Geometry check sheet. Reference: the model listing, model coordinates, mm. Coordinates: 2 decimals unless noted, no trailing zeros. Write each loop counter-clockwise with the first axis right and the second up, starting at its lowest first coordinate (ties: lowest second). Pieces come first, ordered by that corner, then holes. Notation, with made-up numbers: M 12,-39 L 39,-39 A18 ccw 39,-18 Z; hole C 33.5,88.5 d8. An arc over 180 degrees is marked long. Put each result on its own line as item: value. Start each with the question number.
1) Cross-section at B-B on z = 22. Record the cut outline in (x, y).
2) Scan lines: line 1 along X through (y, z) = (-6.5, 29); line 2 along X through (y, z) = (-5.75, 8); line 3 along Z through (x, y) = (1.5, -2.75). Record each from-to range of solid material in increasing order.
3) Gauge pin test, flat ends, axial feed: pin 1 (3 mm diameter, centred on x = 6, y = -5, fed in from +Z); pin 2 (10 mm diameter, centred on y = -4, z = 19.5, fed in from +X); pin 3 (5 mm diameter, centred on x = -1, y = -15, fed in from -Z); pin 4 (6 mm diameter, centred on y = -14, z = 22, fed in from +X). Record the tip position at first contact, or that the pin passes through.
4) Cross-section at A-A on x = -5. Record the cut outline in (y, z), plus the area to 3 significant figures.
from build123d import *

# Parameters (mm, degrees)
F1_DEPTH = 20
F2_R     = 1


# Not quite as in the source:
# - a feature names something its author has since deleted; it is built from what else it names


with BuildPart() as f1:
    # F0 (on Front) → F1 (new body)
    with BuildSketch(Plane.XZ):
        with BuildLine():
            add(Edge.make_bspline(
                [(-14.320673421, 9.4697382301), (-13.2394510975, 9.0805694331), (-11.3333298848, 7.4710466695), (-10.1861008598, 3.0568630532), (-10, 0)],
                knots=[0, 0, 0, 0, 0.3950023229, 1, 1, 1, 1], degree=3))
            Line((-10, 0), (0, 0))
            Line((0, 0), (10, 0))
            add(Edge.make_bspline(
                [(14.320673421, 9.4697382301), (13.2394510975, 9.0805694331), (11.3333298848, 7.4710466695), (10.1861008598, 3.0568630532), (10, 0)],
                knots=[0, 0, 0, 0, 0.3950023229, 1, 1, 1, 1], degree=3))
            Line((14.320673421, 9.4697382301), (0.7904520571, 30))
            add(Edge.make_bspline(
                [(-0.7904520571, 30), (-0.5269680381, 30.1565037668), (0, 30.4695113003), (0.5269680381, 30.1565037668), (0.7904520571, 30)],
                knots=[0, 0, 0, 0, 0.5, 1, 1, 1, 1], degree=3))
            Line((-0.7904520571, 30), (-14.320673421, 9.4697382301))
        make_face()
    extrude(amount=F1_DEPTH)

    # F2
    f2_edges = [f1.edges().sort_by_distance(p)[0] for p in [
        (-14.320673, -10, 9.469738),
        (14.320673, -10, 9.469738),
        (-10.973556, 0, 5.385962),
        (-10.973556, -20, 5.385962),
        (10.973556, 0, 5.385962),
        (10.973556, -20, 5.385962),
    ]]
    fillet(f2_edges, radius=F2_R)


solid = f1.part
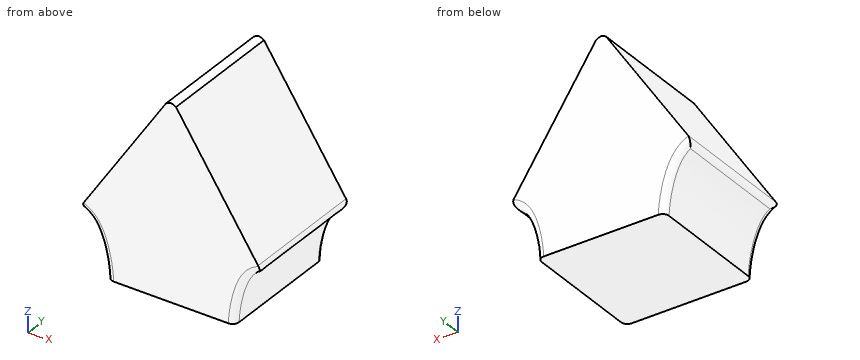
Answer key:
1. outline: M -6.06,-20 L 6.06,-20 L 6.06,0 L -6.06,0 Z
2. line 1: x = -1.45 to 1.45
2. line 2: x = -12.28 to 12.28
2. line 3: z = 0 to 28.92
3. pin 1: stops at z = 24.37
3. pin 2: stops at x = 11.01
3. pin 3: stops at z = 0
3. pin 4: stops at x = 8.04
4. outline: M -20,0 L 0,0 L 0,23.61 L -20,23.61 Z
4. area: 472 mm²
